from build123d import *

# Parameters (mm, degrees)
CROQUIS1_R              = 1.6
SALIENTE_EXTRUIR1_DEPTH = 3


with BuildPart() as part:
    # Croquis1 → Saliente-Extruir1 (new body)
    with BuildSketch(Plane(origin=(0, 0, 0), x_dir=(0, 1, 0), z_dir=(0, 0, 1))):
        with BuildLine():
            Line((0, 6.5), (-17.080114399, 4.058751937))
            ThreePointArc((-17.080114399, 4.058751937), (-20.6, 0), (-17.080114399, -4.058751937))
            Line((-17.080114399, -4.058751937), (0, -6.5))
            Line((0, -6.5), (17.080114399, -4.058751937))
            ThreePointArc((17.080114399, -4.058751937), (20.6, 0), (17.080114399, 4.058751937))
            Line((17.080114399, 4.058751937), (0, 6.5))
        make_face()
        with BuildLine():
            Line((-1.601124605, 1.92), (1.601124605, 1.92))
            ThreePointArc((1.601124605, 1.92), (0, -2.5), (-1.601124605, 1.92))
        make_face(mode=Mode.SUBTRACT)
        with Locations(Location((-16.5, 0, 0), (0, 0, 270))):
            Circle(CROQUIS1_R, mode=Mode.SUBTRACT)
        with Locations(Location((16.5, 0, 0), (0, 0, 270))):
            Circle(CROQUIS1_R, mode=Mode.SUBTRACT)
    extrude(amount=SALIENTE_EXTRUIR1_DEPTH)


solid = part.part
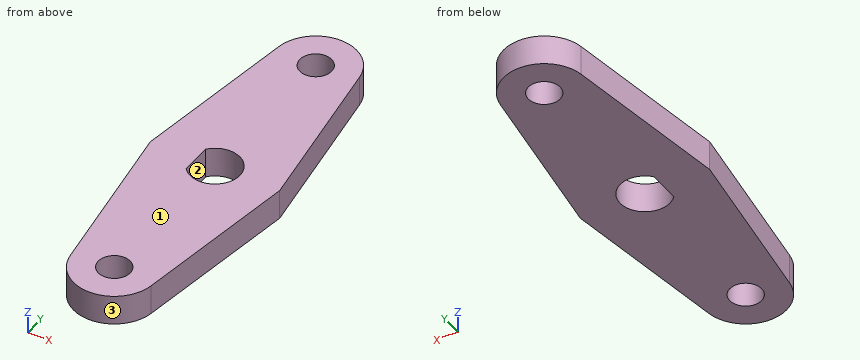
Source: CAD feature listing. Evaluate the final solid. Frame: model axes, mm. Face numbers are marked on the shaded views. Coordinates: 2 decimals unless noted, no trailing zeros. Loops run counter-clockwise (first coordinate to the right, second up) from the corner with the lowest first, then second, coordinate; pieces in that order, holes last. Notation, with made-up numbers: (80, 24.5) - (108, 24.5) arc R21 ccw to (108, 61.5) - close; hole circle Ø3 at (-27.75, -23). An arc over 180 degrees is marked (long way). One line per item, written item: value. Start each with the question number.
1. Mould query, pull axis Y, two halves, no side actions, for the marked faces 1, 2 and 3. Classes: pulls with the +Y half, pulls with the -Y half, needs draft (parallel to the pull), parting line crosses it, or undercut.
2. Section C-C (y = -16.5). Return the cut outline in (x, z).
3. Section D-D (x = -3). Return the cut outline in (y, z).
4. Section A-A (x = 0). Return the cut outline in (y, z), and give its area (3 significant figures).
5. Ray query, L1, parallel to X at y = 0, z = 1.1; L2, parallel to Y at x = 1.25, z = 1.6; L3, parallel to Y at x = -0.5, z = 0.55. Return the intervals inside material, ascending.
6. Section B-B (z = 2). Return the cut outline in (x, y), and give its area (3 significant figures).
7. Contact query for flat-ended pins moving along their axis: P1, Ø1, axis at y = 6, z = 2, coming from the +X side; P2, Ø5, axis at x = 4.5, y = 5.5, coming from the -Z side; P3, Ø2.5, axis at x = 0, y = -16.5, coming from the +Z side. Output: stop coordinate, or through.
Verdict:
1. face 1: needs draft
1. face 2: undercut
1. face 3: pulls with the -Y half
2. outline: (-4.14, 0) - (-1.6, 0) - (-1.6, 3) - (-4.14, 3) - close; (1.6, 0) - (4.14, 0) - (4.14, 3) - (1.6, 3) - close
3. outline: (-19.29, 0) - (19.29, 0) - (19.29, 3) - (-19.29, 3) - close
4. outline: (-20.6, 0) - (-18.1, 0) - (-18.1, 3) - (-20.6, 3) - close; (-14.9, 0) - (-2.5, 0) - (-2.5, 3) - (-14.9, 3) - close; (2.5, 0) - (14.9, 0) - (14.9, 3) - (2.5, 3) - close; (18.1, 0) - (20.6, 0) - (20.6, 3) - (18.1, 3) - close
4. area: 89.4 mm2
5. L1: x = -6.5 to -1.92, 2.5 to 6.5
5. L2: y = -20.4 to -17.5, -15.5 to -2.17, 2.17 to 15.5, 17.5 to 20.4
5. L3: y = -20.57 to -18.02, -14.98 to -2.45, 2.45 to 14.98, 18.02 to 20.57
6. outline: (-6.5, 0) - (-4.06, -17.08) arc R4.1 ccw to (4.06, -17.08) - (6.5, 0) - (4.06, 17.08) arc R4.1 ccw to (-4.06, 17.08) - close; hole (-1.92, -1.6) arc R2.5 ccw (long way) to (-1.92, 1.6) - close; hole circle Ø3.2 at (0, -16.5); hole circle Ø3.2 at (0, 16.5)
6. area: 370 mm2
7. P1: stops at x = 5.71
7. P2: stops at z = 0
7. P3: passes through
